Autodesk Inventor part; units mm, degrees
ref_plane "YZ Plane" through (0, 0, 0) normal (1, 0, 0) x (0, 1, 0)
ref_plane "XZ Plane" through (0, 0, 0) normal (0, 1, 0) x (-1, 0, 0)
ref_plane "XY Plane" through (0, 0, 0) normal (0, 0, 1) x (1, 0, 0)
sketch "Szkic1" plane through (0, 0, 0) normal (0, 1, 0) x (-1, 0, 0)
  line L0 (-25, 55) -> (40, 55)
  line L1 (40, 55) -> (40, -55)
  line L2 (40, -55) -> (-25, -55)
  line L3 (-25, -55) -> (-25, 55)
  point P0 (0, 0)
  point P1 (-25, 0)
  point P2 (40, 0)
  dimension "d0" = 65
  dimension "d1" = 110
  dimension "d2" = 55
  dimension "d25" = 40
extrude "Wyciągnięcie proste1" add sketch "Szkic1" along normal blind 3.5
sketch "Szkic2" plane through (0, 3.5, 0) normal (0, 1, 0) x (1, 0, 0)
  line L0 (12.5, -39.5) -> (-12.5, -39.5)
  line L1 (-12.5, -39.5) -> (-12.5, -34.5)
  line L2 (-12.5, -34.5) -> (12.5, -34.5)
  line L3 (12.5, -34.5) -> (12.5, -39.5)
  point P0 (0, 0)
  point P1 (0, -34.5)
  dimension "d6" = 25
  dimension "d7" = 5
  dimension "d8" = 34.5
  dimension "d9" = 12.5
extrude "Wyciągnięcie proste2" add sketch "Szkic2" along normal blind 70
sketch "Szkic3" plane through (12.5, 3.5, 34.5) normal (0, 0, -1) x (-1, 0, 0)
  circle A0 centre (12.5, 60) radius 4.5
  line L0 (-12.5, 0) -> (52.5, 0)
  line L1 (25, 0) -> (25, 70)
  point P0 (12.5, -3.5)
  dimension "d16" = 9
  dimension "d17" = 60
  dimension "d18" = 12.5
extrude "Wyciągnięcie proste3" cut sketch "Szkic3" against normal up to next
sketch "Szkic4" plane through (0, 3.5, 0) normal (0, 1, 0) x (1, 0, 0)
  line L0 (-32.5, 34.5) -> (17.5, 34.5)
  line L1 (17.5, 34.5) -> (17.5, 39.5)
  line L2 (17.5, 39.5) -> (-32.5, 39.5)
  line L3 (-32.5, 39.5) -> (-32.5, 34.5)
  line L4 (12.5, -34.5) -> (-12.5, -34.5)
  line L5 (25, -55) -> (25, 55)
  point P0 (0, 0)
  point P1 (-7.5, 39.5)
  point P2 (17.5, 37)
  dimension "d22" = 50
  dimension "d23" = 5
  dimension "d24" = 69
  dimension "d26" = 7.5
extrude "Wyciągnięcie proste4" add sketch "Szkic4" along normal blind 90
sketch "Szkic5" plane through (17.5, 3.5, -39.5) normal (0, 0, -1) x (-1, 0, 0)
  line L0 (5, 75) -> (45, 75)
  line L1 (45, 75) -> (45, 55)
  line L2 (45, 55) -> (5, 55)
  line L3 (5, 55) -> (5, 75)
  line L4 (0, 0) -> (0, 90)
  line L5 (-7.5, 0) -> (57.5, 0)
  point P0 (17.5, -3.5)
  point P1 (45, 65)
  dimension "d29" = 40
  dimension "d30" = 20
  dimension "d31" = 5
  dimension "d33" = 65
extrude "Wyciągnięcie proste5" cut sketch "Szkic5" against normal up to next
sketch "Szkic6" plane through (-32.5, 3.5, -39.5) normal (-1, 0, 0) x (0, 0, 1)
  line L0 (-15.5, 0) -> (94.5, 0)
  line L1 (-15.5, 0) -> (0, 26.8468)
  line L2 (-15.5, 0) -> (15.5, 0) construction
  line L3 (0, 0) -> (0, 90)
  line L4 (0, 26.8468) -> (0, 0)
  line L5 (0, 0) -> (-15.5, 0)
  point P0 (39.5, -3.5)
  dimension "d36" = 60
extrude "Wyciągnięcie proste6" add sketch "Szkic6" along normal mid plane 10
sketch "Szkic7" plane through (17.5, 3.5, -34.5) normal (1, 0, 0) x (0, 0, -1)
  line L0 (0, 0) -> (5, 0)
  line L1 (5, 26.8468) -> (20.5, 0)
  line L2 (20.5, 0) -> (5, 26.8468)
  line L3 (5, 26.8468) -> (5, 0)
  line L4 (5, 0) -> (20.5, 0)
  point P0 (-34.5, -3.5)
  point P1 (5, 0)
extrude "Wyciągnięcie proste7" add sketch "Szkic7" along normal mid plane 10
sketch "Szkic8" plane through (12.5, 3.5, 39.5) normal (1, 0, 0) x (0, 0, -1)
  line L0 (-15.5, 0) -> (94.5, 0)
  line L1 (-15.5, 0) -> (0, 26.8468)
  line L2 (-15.5, 0) -> (15.5, 0) construction
  line L3 (0, 0) -> (0, 70)
  line L4 (0, 26.8468) -> (0, 0)
  line L5 (0, 0) -> (-15.5, 0)
  point P0 (39.5, -3.5)
  dimension "d41" = 60
extrude "Wyciągnięcie proste8" add sketch "Szkic8" against normal blind 5
sketch "Szkic9" plane through (-12.5, 3.5, 34.5) normal (-1, 0, 0) x (0, 0, 1)
  line L0 (-89.5, 0) -> (20.5, 0)
  line L1 (20.5, 0) -> (5, 26.8468)
  line L2 (5, 0) -> (5, 70)
  line L3 (20.5, -3.5) -> (20.5, 0)
  line L4 (5, 0) -> (20.5, 0)
  line L5 (5, 0) -> (0, 0)
  line L6 (5, 26.8468) -> (5, 0)
  line L7 (5, 0) -> (20.5, 0)
  point P0 (-34.5, -3.5)
  dimension "d44" = 120
extrude "Wyciągnięcie proste9" add sketch "Szkic9" against normal blind 5
sketch "Szkic10" plane through (0, 3.5, 0) normal (0, 1, 0) x (1, 0, 0)
  line L0 (17.5, 34.5) -> (17.5, 39.5)
  line L1 (17.5, 34.5) -> (22.5, 34.5)
  line L2 (22.5, 34.5) -> (22.5, 39.5)
  line L3 (22.5, 39.5) -> (17.5, 39.5)
  line L4 (17.5, 39.5) -> (17.5, 34.5)
  line L5 (-32.5, 39.5) -> (-32.5, 34.5)
  line L6 (-32.5, 34.5) -> (-37.5, 34.5)
  line L7 (-37.5, 34.5) -> (-37.5, 39.5)
  line L8 (-37.5, 39.5) -> (-32.5, 39.5)
  line L9 (-32.5, 39.5) -> (-32.5, 34.5)
  point P0 (0, 0)
  dimension "d47" = 5
  dimension "d48" = 5
  dimension "d49" = 5
extrude "Wyciągnięcie proste10" add sketch "Szkic10" along normal blind 90
sketch "Szkic11" plane through (12.5, 3.5, 34.5) normal (0, 0, -1) x (-1, 0, 0)
  circle A0 centre (12.5, 60) radius 4.5
  circle A1 centre (12.5, 60) radius 4.5
  line L0 (0, 55) -> (0, 75)
  point P0 (12.5, -3.5)
extrude "Wyciągnięcie proste11" add sketch "Szkic11" against normal blind 5
sketch "Szkic12" plane through (12.5, 3.5, 34.5) normal (0, 0, -1) x (-1, 0, 0)
  circle A0 centre (12.5, 60) radius 5
  line L0 (0, 70) -> (25, 70)
  line L1 (25, 0) -> (25, 70)
  point P0 (12.5, -3.5)
  dimension "d55" = 10
  dimension "d56" = 10
  dimension "d57" = 12.5
extrude "Wyciągnięcie proste12" add sketch "Szkic12" along normal blind 15
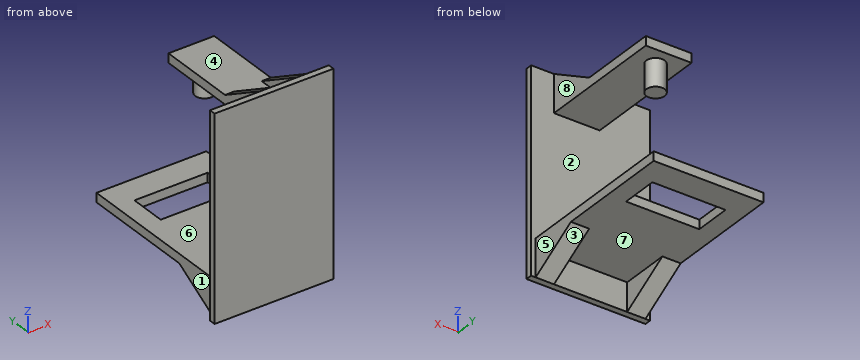
Geometry: final body of the model. Coordinates: model frame, mm. Face numbers are marked on the shaded views. A direction names the side the tool comes from. Coordinates: 2 decimals unless noted, no trailing zeros. Order: outer loops, then holes, each group sorted by start corner. A loop starts at its lowest first (then second) coordinate and runs counter-clockwise, first axis right, second up. Notation, with made-up numbers: (18.5, 43.5) -> (27.5, 43.5) arc R20 cw to (27.5, 63.5) -> close; hole circle Ø2 at (72.25, -22). An arc over 180 degrees is marked (long way). Use CSV: the item, a comma, the result in double quotes.
1) Section A-A on y = 75.5. Output: boundary loops of the cut face in (x, z), then the cut area to 3 significant figures.
Findings:
outline,"(-37.5, -39.5) -> (-27.5, -39.5) -> (-27.5, -34.5) -> (-37.5, -34.5) -> close; (12.5, -39.5) -> (22.5, -39.5) -> (22.5, -34.5) -> (12.5, -34.5) -> close"
area,"100 mm^2"
2) Section C-C on y = 63.5. Output: boundary loops of the cut face in (x, z), then the cut area to 3 significant figures.
Findings:
outline,"(-37.5, -39.5) -> (-27.5, -39.5) -> (-27.5, -34.5) -> (-37.5, -34.5) -> close; (-12.5, 34.5) -> (-5, 34.5) -> (-5, 19.5) -> (5, 19.5) -> (5, 34.5) -> (12.5, 34.5) -> (12.5, 39.5) -> (-12.5, 39.5) -> close; (12.5, -39.5) -> (22.5, -39.5) -> (22.5, -34.5) -> (12.5, -34.5) -> close"
area,"375 mm^2"
3) Pin query (flat end, axial travel): pin 1 Ø1.5 at (y, z) = (47, 41.5) entering from +X; pin 2 Ø8 at (x, y) = (-19, 15) entering from -Z; pin 3 Ø8 at (x, z) = (-6.5, 0.5) entering from +Y; pin 4 Ø5.5 at (x, z) = (-1, 36.5) entering from +Y. Return the tip coordinate at first contact, or that it passes through.
Findings:
pin 1,"passes through"
pin 2,"stops at z = -39.5"
pin 3,"stops at y = 3.5"
pin 4,"stops at y = 73.5"
4) Access query for the marked faces 4, 5, 6, 7 and 8. Directions: +Z, -Z, +X, -X, +Y, -Y. A direction counts if a zero-diameter tool reaches every point of the face in a straight line with its end or side. Return the directions, or none.
Findings:
face 4,"+Z, +Y"
face 5,"+Z, -Z, +X, +Y"
face 6,"+X, -X, +Y"
face 7,"-Z, +Y"
face 8,"+Z, +X, +Y"
5) Section D-D on x = 14.5. Output: boundary loops of the cut face in (y, z), then the cut area to 3 significant figures.
Findings:
outline,"(0, -55) -> (3.5, -55) -> (30.35, -39.5) -> (93.5, -39.5) -> (93.5, -34.5) -> (3.5, -34.5) -> (3.5, 55) -> (0, 55) -> close"
area,"1,040 mm^2"
6) Section B-B on x = 0. Output: boundary loops of the cut face in (y, z), then the cut area to 4 significant figures.
Findings:
outline,"(0, -55) -> (3.5, -55) -> (3.5, -39.5) -> (58.5, -39.5) -> (58.5, -34.5) -> (3.5, -34.5) -> (3.5, 34.5) -> (58.5, 34.5) -> (58.5, 19.5) -> (68.5, 19.5) -> (68.5, 34.5) -> (73.5, 34.5) -> (73.5, 39.5) -> (3.5, 39.5) -> (3.5, 55) -> (0, 55) -> close; (78.5, -39.5) -> (93.5, -39.5) -> (93.5, -34.5) -> (78.5, -34.5) -> close"
area,"1,235 mm^2"
7) Line query: line 1 (X direction, y = 9, z = 46); line 2 (Z direction, x = -9, y = 57); line 3 (Y direction, x = -13, z = -38). Output: solid intervals per line, ascending.
Findings:
line 1,"x = -12.5 to -7.5, 7.5 to 12.5"
line 2,"z = -39.5 to -34.5, 34.5 to 39.5"
line 3,"y = 0 to 58.5, 78.5 to 93.5"
8) Mould query, pull axis Z, two halves, no side actions, for the marked faces 1, 2 and 3. Classes: +Z half, -Z half, draft (parallel to the pull), parting line (faces both ways), or undercut.
Findings:
face 1,"draft"
face 2,"undercut"
face 3,"-Z half"
